Could you check a few things on this model? Use its own coordinates, in mm. A direction names the side the tool comes from. Round coordinates to 2 decimals unless told otherwise and drop trailing zeros. Loops run counter-clockwise (first coordinate to the right, second up) from the corner with the lowest first, then second, coordinate; pieces in that order, holes last. Notation, with made-up numbers: (-16, -12) -> (-3, -12) arc R27 cw to (-3, 26) -> close; hole circle Ø2 at (33, 20). An arc over 180 degrees is marked (long way). Write each question's results on one line, items separated by ' | '.
from build123d import *

# Parameters (mm, degrees)
SKETCH_1_W          = 15
SKETCH_1_H          = 25
EXTRUDE_1_DEPTH     = 1.2
CUT_EXTRUDE_1_REACH = 3.2
SKETCH_2_R          = 1.15
SKETCH_2_W          = 6
SKETCH_2_H          = 2.2
SKETCH_2_W_2        = 2
SKETCH_2_H_2        = 17
SKETCH_3_W          = 2
SKETCH_3_H          = 5
CUT_EXTRUDE_2_DEPTH = 2.2
SKETCH_4_W          = 2
SKETCH_4_H          = 3
CUT_EXTRUDE_3_DEPTH = 2.2


with BuildPart() as part:
    # Эскиз1 → Вытянуть1 (new body)
    with BuildSketch(Plane(origin=(0, 0, 0), x_dir=(0, 0, -1), z_dir=(1, 0, 0))):
        with Locations((7.5, 12.5)):
            Rectangle(SKETCH_1_W, SKETCH_1_H)
    extrude(amount=EXTRUDE_1_DEPTH)

    # Эскиз2 → Вырез-Вытянуть1 (cut, up to next)
    with BuildSketch(Plane(origin=(1.2, 0, 0), x_dir=(0, 0, -1), z_dir=(1, 0, 0)), mode=Mode.PRIVATE) as cut_extrude_1_sk1:
        with Locations((10.7, 2.9)):
            Circle(SKETCH_2_R)
    cut_extrude_1_tool1 = extrude(cut_extrude_1_sk1.sketch, amount=-CUT_EXTRUDE_1_REACH, mode=Mode.PRIVATE) & part.part
    add(cut_extrude_1_tool1.solids().sort_by_distance((1.2, 2.9, -10.7))[0], mode=Mode.SUBTRACT)
    # Эскиз2 → Вырез-Вытянуть1 (cut, up to next)
    with BuildSketch(Plane(origin=(1.2, 0, 0), x_dir=(0, 0, -1), z_dir=(1, 0, 0)), mode=Mode.PRIVATE) as cut_extrude_1_sk2:
        with Locations((2.2, 2.9)):
            Circle(SKETCH_2_R)
    cut_extrude_1_tool2 = extrude(cut_extrude_1_sk2.sketch, amount=-CUT_EXTRUDE_1_REACH, mode=Mode.PRIVATE) & part.part
    add(cut_extrude_1_tool2.solids().sort_by_distance((1.2, 2.9, -2.2))[0], mode=Mode.SUBTRACT)
    # Эскиз2 → Вырез-Вытянуть1 (cut, up to next)
    with BuildSketch(Plane(origin=(1.2, 0, 0), x_dir=(0, 0, -1), z_dir=(1, 0, 0)), mode=Mode.PRIVATE) as cut_extrude_1_sk3:
        with Locations((3, 23.9)):
            Rectangle(SKETCH_2_W, SKETCH_2_H)
    cut_extrude_1_tool3 = extrude(cut_extrude_1_sk3.sketch, amount=-CUT_EXTRUDE_1_REACH, mode=Mode.PRIVATE) & part.part
    add(cut_extrude_1_tool3.solids().sort_by_distance((1.2, 23.9, -3))[0], mode=Mode.SUBTRACT)
    # Эскиз2 → Вырез-Вытянуть1 (cut, up to next)
    with BuildSketch(Plane(origin=(1.2, 0, 0), x_dir=(0, 0, -1), z_dir=(1, 0, 0)), mode=Mode.PRIVATE) as cut_extrude_1_sk4:
        with BuildLine():
            Line((5, 6), (9, 6))
            ThreePointArc((9, 6), (10, 7), (9, 8))
            Line((9, 8), (9, 19))
            ThreePointArc((9, 19), (10, 20), (9, 21))
            Line((9, 21), (5, 21))
            ThreePointArc((5, 21), (4, 20), (5, 19))
            Line((5, 19), (5, 8))
            ThreePointArc((5, 8), (4, 7), (5, 6))
        make_face()
    cut_extrude_1_tool4 = extrude(cut_extrude_1_sk4.sketch, amount=-CUT_EXTRUDE_1_REACH, mode=Mode.PRIVATE) & part.part
    add(cut_extrude_1_tool4.solids().sort_by_distance((1.2, 13.5, -7))[0], mode=Mode.SUBTRACT)
    # Эскиз2 → Вырез-Вытянуть1 (cut, up to next)
    with BuildSketch(Plane(origin=(1.2, 0, 0), x_dir=(0, 0, -1), z_dir=(1, 0, 0)), mode=Mode.PRIVATE) as cut_extrude_1_sk5:
        with Locations((14, 13.5)):
            Rectangle(SKETCH_2_W_2, SKETCH_2_H_2)
    cut_extrude_1_tool5 = extrude(cut_extrude_1_sk5.sketch, amount=-CUT_EXTRUDE_1_REACH, mode=Mode.PRIVATE) & part.part
    add(cut_extrude_1_tool5.solids().sort_by_distance((1.2, 13.5, -14))[0], mode=Mode.SUBTRACT)

    # Эскиз3 → Вырез-Вытянуть2 (cut, through all)
    with BuildSketch(Plane(origin=(1.2, 0, 0), x_dir=(0, 0, -1), z_dir=(1, 0, 0))):
        with Locations((14, 2.5)):
            Rectangle(SKETCH_3_W, SKETCH_3_H)
    extrude(amount=-CUT_EXTRUDE_2_DEPTH, mode=Mode.SUBTRACT)

    # Эскиз4 → Вырез-Вытянуть3 (cut, through all)
    with BuildSketch(Plane(origin=(1.2, 0, 0), x_dir=(0, 0, -1), z_dir=(1, 0, 0))):
        with Locations((14, 23.5)):
            Rectangle(SKETCH_4_W, SKETCH_4_H)
    extrude(amount=-CUT_EXTRUDE_3_DEPTH, mode=Mode.SUBTRACT)


solid = part.part
1) I want a section at A-A, the plane z = -6.5. Write out the boundary of the cut face in (x, y), plus the area to 3 significant figures.
Model answer:
outline: (0, 0) -> (1.2, 0) -> (1.2, 6) -> (0, 6) -> close; (0, 21) -> (1.2, 21) -> (1.2, 25) -> (0, 25) -> close | area: 12.0 mm2
2) I want a section at B-B, the plane y = 15. Write out the boundary of the cut face in (x, z).
Model answer:
outline: (0, -13) -> (1.2, -13) -> (1.2, -9) -> (0, -9) -> close; (0, -5) -> (1.2, -5) -> (1.2, 0) -> (0, 0) -> close
3) For faces 4 (the flat face through (1, 24, -6)), 5 (the flat face through (1, 25, -9)), 6 (the cylindrical face through (1, 7, -10)), which set-ups out of +Z, -Z, +X, -X, +Y, -Y let a thin tool reach every point of the face, with its end or its side?
Model answer:
face 4: +Z, +X, -X, +Y | face 5: +Z, -Z, +X, -X, +Y | face 6: +X, -X
4) I need wall thicknesses on line 1 (Y direction, x = 0.55, z = -2.2); line 2 (Z direction, x = 0.9, y = 14.25); line 3 (Y direction, x = 0.7, z = -7.5). Which ranges of each line are inside material? Lowest first, please.
Model answer:
line 1: y = 0 to 1.75, 4.05 to 22.8 | line 2: z = -13 to -9, -5 to 0 | line 3: y = 0 to 6, 21 to 25
5) I want a section at C-C, the plane x = 0.55. Write out the boundary of the cut face in (y, z).
Model answer:
outline: (0, -13) -> (25, -13) -> (25, -6) -> (22.8, -6) -> (22.8, 0) -> (0, 0) -> close; hole circle Ø2.3 at (2.9, -10.7); hole circle Ø2.3 at (2.9, -2.2); hole (6, -9) arc R1 ccw to (8, -9) -> (19, -9) arc R1 ccw to (21, -9) -> (21, -5) arc R1 ccw to (19, -5) -> (8, -5) arc R1 ccw to (6, -5) -> close
6) If we mould it in two halves opening along Z, with no side actions, what happens to faces 1 (the flat face through (1, 6, -7)), 2 (the flat face through (1.2, 12.7, -9.3)), 3 (the flat face through (1, 12, -13))? For each: released by +Z, released by -Z, zero draft, split by the parting line, or undercut.
Model answer:
face 1: undercut | face 2: zero draft | face 3: released by -Z
7) I want a section at D-D, the plane y = 2.9. Write out the boundary of the cut face in (x, z).
Model answer:
outline: (0, -13) -> (1.2, -13) -> (1.2, -11.85) -> (0, -11.85) -> close; (0, -9.55) -> (1.2, -9.55) -> (1.2, -3.35) -> (0, -3.35) -> close; (0, -1.05) -> (1.2, -1.05) -> (1.2, 0) -> (0, 0) -> close
8) I'm going to push flat-ended pins straight in: pin 1 (0.6 mm diameter, centred on x = 0.5, y = 24, fed in from +Z); pin 2 (1.4 mm diameter, centred on y = 2.9, z = -2.2, fed in from +X). Where does each tip first touch, or does it pass through?
Model answer:
pin 1: stops at z = -6 | pin 2: passes through
